For this review, take the finished solid that the model builds, in its own axes (mm). Round coordinates to 2 decimals unless told otherwise and drop trailing zeros. Order: outer loops, then holes, each group sorted by start corner. A loop starts at its lowest first (then second) coordinate and runs counter-clockwise, first axis right, second up. Notation, with made-up numbers: M 6.5,17 L 64.5,17 A18 cw 64.5,47 Z; hole C 64,77.25 d5. An arc over 180 degrees is marked long. Use a Markdown table: item, result.
from build123d import *

# Parameters (mm, degrees)
SKETCH_1_W          = 55
SKETCH_1_H          = 34.996183206
EXTRUDE_1_DEPTH     = 3
CHAMFER_1_SIZE      = 9.5
FILLET_1_R          = 3
SKETCH_2_R          = 1.65
CUT_EXTRUDE_1_DEPTH = 4


with BuildPart() as part:
    # 草图1 → 凸台-拉伸1 (new body)
    with BuildSketch(Plane.XY):
        Rectangle(SKETCH_1_W, SKETCH_1_H)
    extrude(amount=EXTRUDE_1_DEPTH)

    # 倒角1
    chamfer_1_edges = [part.edges().sort_by_distance(p)[0] for p in [
        (27.5, -17.498091603, 1.5),
        (-27.5, -17.498091603, 1.5),
        (-27.5, 17.498091603, 1.5),
        (27.5, 17.498091603, 1.5),
    ]]
    chamfer(chamfer_1_edges, length=CHAMFER_1_SIZE)

    # 圆角1
    fillet_1_edges = [part.edges().sort_by_distance(p)[0] for p in [
        (-27.5, -7.998091603, 1.5),
        (-27.5, 7.998091603, 1.5),
        (18, 17.498091603, 1.5),
        (-18, 17.498091603, 1.5),
        (18, -17.498091603, 1.5),
        (-18, -17.498091603, 1.5),
        (27.5, 7.998091603, 1.5),
        (27.5, -7.998091603, 1.5),
    ]]
    fillet(fillet_1_edges, radius=FILLET_1_R)

    # 草图2 → 切除-拉伸1 (cut, through all)
    with BuildSketch(Plane.XY.offset(3)):
        with Locations((-21.5, 0)):
            Circle(SKETCH_2_R)
        with Locations((21.5, 0)):
            Circle(SKETCH_2_R)
    extrude(amount=-CUT_EXTRUDE_1_DEPTH, mode=Mode.SUBTRACT)


solid = part.part
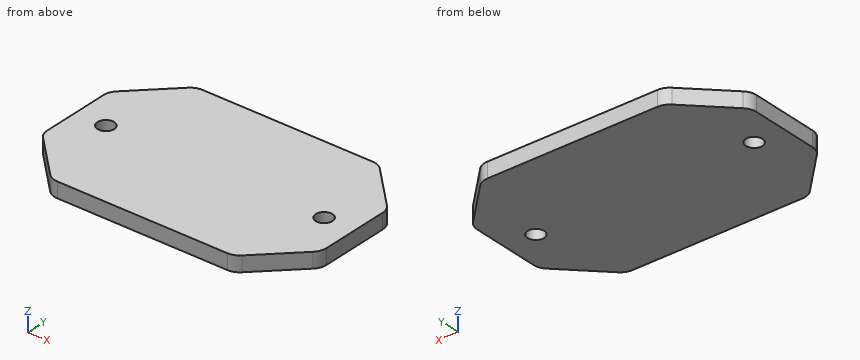
Q1. Add section C-C (x = -21.5). Write out the cut boundary in (y, z).
Determined:
| item | result |
|---|---|
| outline | M -14,0 L -1.65,0 L -1.65,3 L -14,3 Z; M 1.65,0 L 14,0 L 14,3 L 1.65,3 Z |
Q2. Add section D-D (y = 14). Write out the cut boundary in (x, z).
Determined:
| item | result |
|---|---|
| outline | M -21.5,0 L 21.5,0 L 21.5,3 L -21.5,3 Z |
Q3. Add section B-B (z = 1.95). Write out the cut boundary in (x, y).
Determined:
| item | result |
|---|---|
| outline | M -27.5,-6.76 A3 ccw -26.62,-8.88 L -18.88,-16.62 A3 ccw -16.76,-17.5 L 16.76,-17.5 A3 ccw 18.88,-16.62 L 26.62,-8.88 A3 ccw 27.5,-6.76 L 27.5,6.76 A3 ccw 26.62,8.88 L 18.88,16.62 A3 ccw 16.76,17.5 L -16.76,17.5 A3 ccw -18.88,16.62 L -26.62,8.88 A3 ccw -27.5,6.76 Z; hole C -21.5,0 d3.3; hole C 21.5,0 d3.3 |
Q4. Clearance check with flat-ended pins moving along their axes: pin 1 (3 mm diameter, centred on x = -21.5, y = 0, fed in from +Z); pin 2 (5.5 mm diameter, centred on x = 21.5, y = 0, fed in from +Z). State where each tip first meets the part, or that it passes through.
Determined:
| item | result |
|---|---|
| pin 1 | passes through |
| pin 2 | stops at z = 3 |
Q5. Wall thickness on line 1 along Y through (x, z) = (-21.5, 2.45); line 2 along Y through (x, z) = (17, 1.2); line 3 along Y through (x, z) = (18, 0.9): over which ranges is each line inside the solid? List them lowest first. Write a range as [from, to].
Determined:
| item | result |
|---|---|
| line 1 | y = [-14, -1.65], [1.65, 14] |
| line 2 | y = [-17.49, 17.49] |
| line 3 | y = [-17.23, 17.23] |
Q6. Add section A-A (y = 0). Write out the cut boundary in (x, z).
Determined:
| item | result |
|---|---|
| outline | M -27.5,0 L -23.15,0 L -23.15,3 L -27.5,3 Z; M -19.85,0 L 19.85,0 L 19.85,3 L -19.85,3 Z; M 23.15,0 L 27.5,0 L 27.5,3 L 23.15,3 Z |
